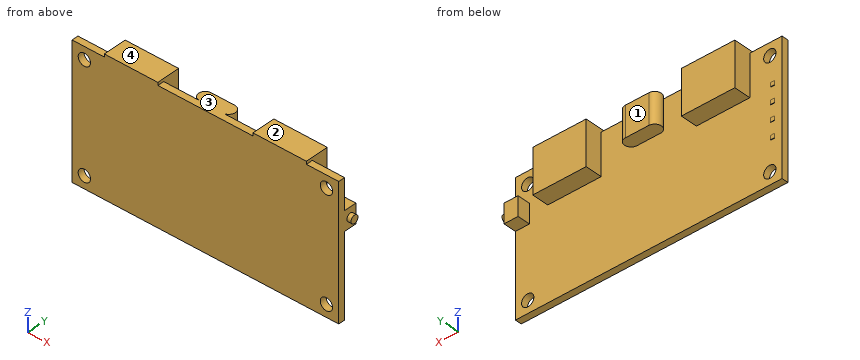
Autodesk Inventor part; units mm, degrees
ref_plane "YZ Plane" through (0, 0, 0) normal (1, 0, 0) x (0, 1, 0)
ref_plane "XZ Plane" through (0, 0, 0) normal (0, 1, 0) x (-1, 0, 0)
ref_plane "XY Plane" through (0, 0, 0) normal (0, 0, 1) x (1, 0, 0)
sketch "草圖1" plane through (0, 0, 0) normal (0, 1, 0) x (-1, 0, 0)
  line L0 (0, 0) -> (-65, 0)
  line L1 (-65, 0) -> (-65, -32.3)
  line L2 (-65, -32.3) -> (0, -32.3)
  line L3 (0, -32.3) -> (0, 0)
  circle A0 centre (-3, -3) radius 1.5
  circle A1 centre (-3, -29.3) radius 1.5
  circle A2 centre (-62, -3) radius 1.5
  circle A3 centre (-62, -29.3) radius 1.5
  dimension "d0" = 65
  dimension "d1" = 32.3
  dimension "d4" = 3
  dimension "d5" = 3
  dimension "d6" = 3
  dimension "d7" = 3
  dimension "d8" = 3
  dimension "d9" = 3
  dimension "d10" = 3
  dimension "d11" = 3
  dimension "d12" = 3
  dimension "d13" = 3
  dimension "d14" = 3
  dimension "d15" = 3
extrude "擠出1" add sketch "草圖1" along normal blind 1.6
sketch "草圖2" plane through (0, 0, 0) normal (0, 0, 1) x (1, 0, 0)
  line L0 (0, 0) -> (65, 0)
  line L1 (65, 0) -> (65, 1.6)
  line L2 (0, 1.6) -> (65, 1.6)
  line L3 (0, 0) -> (0, 1.6)
  line L4 (7.88, 0) -> (20.91, 0)
  line L5 (20.91, 0) -> (20.91, 5.7)
  line L6 (20.91, 5.7) -> (7.88, 5.7)
  line L7 (7.88, 5.7) -> (7.88, 0)
  line L8 (44.09, 0) -> (57.12, 0)
  line L9 (57.12, 0) -> (57.12, 5.7)
  line L10 (57.12, 5.7) -> (44.09, 5.7)
  line L11 (44.09, 5.7) -> (44.09, 0)
  point P0 (44.09, 1.6)
  point P1 (57.12, 1.6)
  dimension "d16" = 13.03
  dimension "d17" = 5.7
  dimension "d18" = 13.03
  dimension "d19" = 5.7
  dimension "d20" = 7.88
  dimension "d21" = 7.88
extrude "擠出2" add sketch "草圖2" along normal blind 0.7 contours L7 L2 L5 L0 | L7 L6 L5 L2 | L11 L2 L9 L0 | L11 L10 L9 L2
sketch "草圖3" plane through (0, 0, 0) normal (0, 0, -1) x (-1, 0, 0)
  line L0 (-7.88, 1.6) -> (-20.91, 1.6)
  line L1 (-7.88, 5.7) -> (-7.88, 1.6)
  line L2 (-20.91, 5.7) -> (-7.88, 5.7)
  line L3 (-20.91, 1.6) -> (-20.91, 5.7)
  line L4 (-57.12, 5.7) -> (-44.09, 5.7)
  line L5 (-44.09, 5.7) -> (-44.09, 1.6)
  line L6 (-57.12, 5.7) -> (-44.09, 5.7)
  line L7 (-57.12, 1.6) -> (-57.12, 5.7)
  line L8 (-7.88, 1.6) -> (-20.91, 1.6)
  line L9 (-7.88, 5.7) -> (-7.88, 1.6)
  line L10 (-20.91, 5.7) -> (-7.88, 5.7)
  line L11 (-20.91, 1.6) -> (-20.91, 5.7)
  line L12 (-44.09, 1.6) -> (-57.12, 1.6)
  point P0 (0, 0)
extrude "擠出3" add sketch "草圖3" along normal blind 10.1
sketch "草圖4" plane through (65, 0, 0) normal (0, 0, 1) x (1, 0, 0)
  line L0 (-44.09, 1.6) -> (-44.09, 0)
  line L1 (-65, 0) -> (-57.12, 0)
  line L2 (0, 0) -> (0, 1.6)
  line L3 (-7.88, 1.6) -> (0, 1.6)
  line L4 (-65, 1.6) -> (-57.12, 1.6)
  line L5 (-44.09, 1.6) -> (-20.91, 1.6)
  line L6 (-35.37, 1.6) -> (-29.63, 1.6)
  line L7 (-28.03, 3.2) -> (-28.03, 3.2)
  line L8 (-29.63, 4.8) -> (-35.37, 4.8)
  line L9 (-36.97, 3.2) -> (-36.97, 3.2)
  arc A0 (-35.37, 4.8) -> (-36.97, 3.2) centre (-35.37, 3.2) ccw
  arc A1 (-36.97, 3.2) -> (-35.37, 1.6) centre (-35.37, 3.2) ccw
  arc A2 (-29.63, 1.6) -> (-28.03, 3.2) centre (-29.63, 3.2) ccw
  arc A3 (-28.03, 3.2) -> (-29.63, 4.8) centre (-29.63, 3.2) ccw
  line L10 (0, 0) -> (-65, 0)
  line L11 (-57.12, 0) -> (-57.12, 1.6)
  line L12 (-65, 0) -> (-65, 1.6)
  line L13 (-44.09, 0) -> (-20.91, 0)
  line L14 (-20.91, 0) -> (-20.91, 1.6)
  line L15 (-7.88, 1.6) -> (-7.88, 0)
  line L16 (-7.88, 0) -> (0, 0)
  point P0 (-36.97, 1.6)
  point P1 (-28.03, 4.8)
  point P2 (-28.03, 1.6)
  point P3 (-36.97, 4.8)
  point P4 (-32.5, 4.8)
  point P5 (-32.5, 0)
  point P6 (-35.37, 1.6)
  point P7 (-29.63, 1.6)
  dimension "d26" = 8.94
  dimension "d27" = 3.2
  dimension "d28" = 1.6
extrude "擠出4" add sketch "草圖4" against normal blind 7.4 contours A1 A0 L8 A3 A2 L5
sketch "草圖5" plane through (65, 0, 0) normal (1, 0, 0) x (0, 0, -1)
  line L0 (0, 0) -> (32.3, 0)
  line L1 (32.3, 0) -> (32.3, 1.6)
  line L2 (0, 1.6) -> (32.3, 1.6)
  line L3 (0, 0) -> (0, 1.6)
  line L4 (7.5, 1.6) -> (12.2, 1.6)
  line L5 (12.2, 1.6) -> (12.2, 4.7)
  line L6 (12.2, 4.7) -> (7.5, 4.7)
  line L7 (7.5, 4.7) -> (7.5, 1.6)
  dimension "d31" = 4.7
  dimension "d32" = 3.1
  dimension "d33" = 7.5
extrude "擠出5" add sketch "草圖5" against normal blind 3.4 contours L7 L6 L5 L2
sketch "草圖6" plane through (65, 0, 0) normal (1, 0, 0) x (0, 0, -1)
  line L0 (0, 0) -> (32.3, 0)
  line L1 (32.3, 0) -> (32.3, 1.6)
  line L2 (12.2, 1.6) -> (32.3, 1.6)
  line L3 (12.2, 1.6) -> (12.2, 4.7)
  line L4 (12.2, 4.7) -> (7.5, 4.7)
  line L5 (7.5, 4.7) -> (7.5, 1.6)
  line L6 (0, 1.6) -> (7.5, 1.6)
  line L7 (0, 0) -> (0, 1.6)
  line L8 (7.5, 1.6) -> (12.2, 1.6)
  circle A0 centre (9.85, 3.19) radius 0.95
  dimension "d36" = 1.9
extrude "擠出6" add sketch "草圖6" along normal blind 1 contours A0
sketch "草圖7" plane through (0, 1.6, 0) normal (0, 1, 0) x (1, 0, 0)
  circle A0 centre (62, 29.3) radius 1.5
  circle A1 centre (62, 3) radius 1.5
  circle A2 centre (3, 29.3) radius 1.5
  circle A3 centre (3, 3) radius 1.5
  line L0 (65, 7.5) -> (61.6, 7.5)
  line L1 (61.6, 7.5) -> (61.6, 12.2)
  line L2 (61.6, 12.2) -> (65, 12.2)
  line L3 (65, 12.2) -> (65, 32.3)
  line L4 (65, 32.3) -> (0, 32.3)
  line L5 (0, 32.3) -> (0, 0)
  line L6 (0, 0) -> (7.88, 0)
  line L7 (7.88, 0) -> (7.88, 10.1)
  line L8 (7.88, 10.1) -> (20.91, 10.1)
  line L9 (20.91, 10.1) -> (20.91, 0)
  line L10 (20.91, 0) -> (29.63, 0)
  line L11 (29.63, 0) -> (29.63, 7.4)
  line L12 (29.63, 7.4) -> (35.37, 7.4)
  line L13 (35.37, 0) -> (35.37, 7.4)
  line L14 (35.37, 0) -> (44.09, 0)
  line L15 (44.09, 0) -> (44.09, 10.1)
  line L16 (44.09, 10.1) -> (57.12, 10.1)
  line L17 (57.12, 10.1) -> (57.12, 0)
  line L18 (57.12, 0) -> (65, 0)
  line L19 (65, 0) -> (65, 7.5)
  line L20 (1.8, 22.24) -> (2.8, 22.24)
  line L21 (2.8, 22.24) -> (2.8, 21.24)
  line L22 (2.8, 21.24) -> (1.8, 21.24)
  line L23 (1.8, 21.24) -> (1.8, 22.24)
  line L24 (1.8, 22.24) -> (2.8, 21.24) construction
  line L25 (2.8, 22.24) -> (1.8, 21.24) construction
  line L26 (1.8, 10.24) -> (2.8, 10.24)
  line L27 (2.8, 10.24) -> (2.8, 9.24)
  line L28 (2.8, 9.24) -> (1.8, 9.24)
  line L29 (1.8, 9.24) -> (1.8, 10.24)
  line L30 (1.8, 10.24) -> (2.8, 9.24) construction
  line L31 (2.8, 10.24) -> (1.8, 9.24) construction
  line L32 (1.8, 14.24) -> (2.8, 14.24)
  line L33 (2.8, 14.24) -> (2.8, 13.24)
  line L34 (2.8, 13.24) -> (1.8, 13.24)
  line L35 (1.8, 13.24) -> (1.8, 14.24)
  line L36 (1.8, 14.24) -> (2.8, 13.24) construction
  line L37 (2.8, 14.24) -> (1.8, 13.24) construction
  line L38 (1.8, 17.24) -> (2.8, 17.24)
  line L39 (2.8, 17.24) -> (2.8, 18.24)
  line L40 (2.8, 18.24) -> (1.8, 18.24)
  line L41 (1.8, 18.24) -> (1.8, 17.24)
  line L42 (1.8, 17.24) -> (2.8, 18.24) construction
  line L43 (2.8, 17.24) -> (1.8, 18.24) construction
  point P0 (2.3, 21.74)
  point P1 (2.3, 9.74)
  point P2 (2.3, 13.74)
  point P3 (2.3, 17.74)
  point P4 (2.3, 17.24)
  dimension "d39" = 1
  dimension "d40" = 1
  dimension "d41" = 1
  dimension "d42" = 1
  dimension "d43" = 1
  dimension "d44" = 1
  dimension "d45" = 1
  dimension "d46" = 1
  dimension "d47" = 2.3
  dimension "d48" = 10.56
  dimension "d55" = 4
  dimension "d56" = 4
  dimension "d57" = 4
extrude "擠出7" add sketch "草圖7" along normal blind 0.1 contours L20 L21 L22 L23 | L26 L27 L28 L29 | L32 L33 L34 L35 | L41 L40 L39 L38
equation "\"d18\" = d16"
equation "\"d19\" = d17"
equation "\"d21\" = d20"
properties part number "circuit board"
Model file for the job. Use its own axes, mm. Face numbers are marked on the shaded views. A direction names the side the tool comes from. Give positions to 0.01 mm unless a question says otherwise; leave off trailing zeros. Write each loop counter-clockwise with the first axis right and the second up, starting at its lowest first coordinate (ties: lowest second). Pieces come first, ordered by that corner, then holes. Notation, with made-up numbers: M 19.25,82.25 L 41.25,82.25 A17 ccw 41.25,102.25 Z; hole C 49,-9 d2. An arc over 180 degrees is marked long. Use a Markdown table: item, result.
1) Pull direction X, two halves, no side cores. Call the marked faces 3 and 4: +X half, -X half, draft (parallel to the pull), parting line (faces both ways), or undercut.
Responses:
| item | result |
|---|---|
| face 3 | undercut |
| face 4 | draft |
2) Tool access for the marked faces 1 and 2: list every direction of +Z, -Z, +X, -X, +Y, -Y with a clear straight run to the whole face (end or side of a thin tool).
Responses:
| item | result |
|---|---|
| face 1 | +Z, -Z, +Y |
| face 2 | +Z, +X, -X, +Y, -Y |
3) Pin check, flat tips, straight feed: pin 1 (3 mm diameter, centred on y = 4, z = -6, fed in from -X); pin 2 (3 mm diameter, centred on x = 39, z = -3, fed in from +Y); pin 3 (6 mm diameter, centred on x = 31, z = -8, fed in from +Y). Stop position of each tip, or through.
Responses:
| item | result |
|---|---|
| pin 1 | stops at x = 7.88 |
| pin 2 | stops at y = 1.6 |
| pin 3 | stops at y = 4.8 |
4) Cut at C-C (x = 14). List the corners of the cut face in (y, z), and give its area (3 significant figures).
Responses:
| item | result |
|---|---|
| outline | M 0,-32.3 L 1.6,-32.3 L 1.6,-10.1 L 5.7,-10.1 L 5.7,0.7 L 0,0.7 Z |
| area | 97.1 mm2 |
5) Cut at D-D (z = -11.5). List the corners of the cut face in (x, y).
Responses:
| item | result |
|---|---|
| outline | M 0,0 L 65,0 L 65,4.7 L 61.6,4.7 L 61.6,1.6 L 0,1.6 Z |
6) Drill centre lines: line 1 (Z direction, x = 3, y = 0.9); line 2 (X direction, y = 2, z = -2.5); line 3 (Y direction, x = 16, z = -25.5). Where is each one in solid material? Low to high. Write a range as from..to.
Responses:
| item | result |
|---|---|
| line 1 | z = -32.3..-30.8, -27.8..-4.5, -1.5..0 |
| line 2 | x = 7.88..20.91, 28.57..36.43, 44.09..57.12 |
| line 3 | y = 0..1.6 |
7) Cut at B-B (y = 0.95). List the corners of the cut face in (x, z).
Responses:
| item | result |
|---|---|
| outline | M 0,-32.3 L 65,-32.3 L 65,0 L 57.12,0 L 57.12,0.7 L 44.09,0.7 L 44.09,0 L 20.91,0 L 20.91,0.7 L 7.88,0.7 L 7.88,0 L 0,0 Z; hole C 3,-29.3 d3; hole C 3,-3 d3; hole C 62,-29.3 d3; hole C 62,-3 d3 |
8) Cut at A-A (z = -29.3). List the corners of the cut face in (x, y), and give its area (3 significant figures).
Responses:
| item | result |
|---|---|
| outline | M 0,0 L 1.5,0 L 1.5,1.6 L 0,1.6 Z; M 4.5,0 L 60.5,0 L 60.5,1.6 L 4.5,1.6 Z; M 63.5,0 L 65,0 L 65,1.6 L 63.5,1.6 Z |
| area | 94.4 mm2 |
